```python
from build123d import *

# Parameters (mm, degrees)
SKETCH1_R                = 57.15
SKETCH1_R_2              = 53.34
SCHEDULED_CHAMBER_DEPTH  = 260.35
SKETCH2_R                = 76.2
SKETCH2_R_2              = 57.15
FLANGE_DEPTH             = 6.35
ORIGINAL_BOLT_HOLE_REACH = 283.771
SKETCH3_R                = 3.175
BOLT_HOLE_PATTERN_COUNT  = 8


with BuildPart() as part:
    # Sketch1 → Scheduled Chamber (new body)
    with BuildSketch(Plane(origin=(0, 0, 0), x_dir=(1, 0, 0), z_dir=(0, 1, 0))):
        with Locations(Location((0, 0, 0), (0, 0, 270))):
            Circle(SKETCH1_R)
        with Locations(Location((0, 0, 0), (0, 0, 270))):
            Circle(SKETCH1_R_2, mode=Mode.SUBTRACT)
    extrude(amount=-SCHEDULED_CHAMBER_DEPTH)

    # Sketch2 → Flange (add)
    with BuildSketch(Plane(origin=(0, 0, 0), x_dir=(1, 0, 0), z_dir=(0, 1, 0))):
        with Locations(Location((0, 0, 0), (0, 0, 270))):
            Circle(SKETCH2_R)
        with Locations(Location((0, 0, 0), (0, 0, 270))):
            Circle(SKETCH2_R_2, mode=Mode.SUBTRACT)
    extrude(amount=-FLANGE_DEPTH)

    # Sketch3 → Original Bolt Hole (cut, up to next)
    with BuildSketch(Plane(origin=(0, 0, 0), x_dir=(1, 0, 0), z_dir=(0, 1, 0)), mode=Mode.PRIVATE) as original_bolt_hole_sk1:
        with Locations(Location((0, 64.77, 0), (0, 0, 270))):
            Circle(SKETCH3_R)
    original_bolt_hole_tool1 = extrude(original_bolt_hole_sk1.sketch, amount=-ORIGINAL_BOLT_HOLE_REACH, mode=Mode.PRIVATE) & part.part
    original_bolt_hole = original_bolt_hole_tool1.solids().sort_by_distance((0, 0, -64.77))[0]
    add(original_bolt_hole, mode=Mode.SUBTRACT)

    # Bolt Hole Pattern: Original Bolt Hole ×8 about axis
    bolt_hole_pattern_axis = Axis((0, 0, 0), (0, 1, 0))
    for i in range(1, BOLT_HOLE_PATTERN_COUNT):
        add(original_bolt_hole.rotate(bolt_hole_pattern_axis, i * 360 / BOLT_HOLE_PATTERN_COUNT), mode=Mode.SUBTRACT)


solid = part.part
```
Here's how the part is built. I have some questions about the finished solid (model axes, mm). A direction names the side the tool comes from. Round coordinates to 2 decimals unless told otherwise and drop trailing zeros. Order: outer loops, then holes, each group sorted by start corner. A loop starts at its lowest first (then second) coordinate and runs counter-clockwise, first axis right, second up. Notation, with made-up numbers: M 54,46 L 111,46 A19 ccw 111,80 Z; hole C -8.5,-39.75 d7. An arc over 180 degrees is marked long. Use CSV: the item, a comma, the result in double quotes.
1) I want a section at C-C (z = 64.77). List the corners of the cut face in (x, y) for me (3 decimals), then the cut area to 3 significant figures.
Taken from the geometry:
outline,"M -40.141,-6.35 L -3.175,-6.35 L -3.175,0 L -40.141,0 Z; M 3.175,-6.35 L 40.141,-6.35 L 40.141,0 L 3.175,0 Z"
area,"469 mm^2"
2) If we mould it in two halves opening along Z, with no side actions, what happens to faces 1 (the flat face through (51, -6.35, -29)), 2 (the cylindrical face through (-46.367, -3.131, -60.47)), 3 (the cylindrical face through (44.585, -3.131, 42.866))? For each: pulls with the +Z half, pulls with the -Z half, needs draft (parallel to the pull), parting line crosses it, or undercut.
Taken from the geometry:
face 1,"needs draft"
face 2,"parting line crosses it"
face 3,"undercut"
3) I need wall thicknesses on line 1 along X through (y, z) = (-29, -2) (1 decimal); line 2 along X through (y, z) = (-147.5, -6.5); line 3 along Z through (x, y) = (36.5, -83). Which ranges of each line are inside material? Lowest first, please. Write a range as [from, to].
Taken from the geometry:
line 1,"[-57.1, -53.3], [53.3, 57.1]"
line 2,"[-56.78, -52.94], [52.94, 56.78]"
line 3,"[-43.98, -38.9], [38.9, 43.98]"
4) I want a section at D-D (y = -176.5). List the corners of the cut face in (x, z) for me, then the cut area to 3 significant figures.
Taken from the geometry:
outline,"C 0,0 d114.3; hole C 0,0 d106.68"
area,"1,320 mm^2"
5) I want a section at B-B (x = -64.77). List the corners of the cut face in (y, z) for me (3 decimals).
Taken from the geometry:
outline,"M -6.35,-40.141 L 0,-40.141 L 0,-3.175 L -6.35,-3.175 Z; M -6.35,3.175 L 0,3.175 L 0,40.141 L -6.35,40.141 Z"
6) I want a section at A-A (z = 0). List the corners of the cut face in (x, y) for me (3 decimals), then the cut area to 3 significant figures.
Taken from the geometry:
outline,"M -76.2,-6.35 L -67.945,-6.35 L -67.945,0 L -76.2,0 Z; M -61.595,-6.35 L -57.15,-6.35 L -57.15,-260.35 L -53.34,-260.35 L -53.34,0 L -61.595,0 Z; M 53.34,-260.35 L 57.15,-260.35 L 57.15,-6.35 L 61.595,-6.35 L 61.595,0 L 53.34,0 Z; M 67.945,-6.35 L 76.2,-6.35 L 76.2,0 L 67.945,0 Z"
area,"2,150 mm^2"
7) I'm going to push flat-ended pins straight in: P1, Ø10, axis at x = -45.8, z = -45.8, coming from the -Y side; P2, Ø5, axis at x = 64.77, z = 0, coming from the +Y side; P3, Ø6, axis at y = -92.5, z = -28, coming from the +X side; P4, Ø1.5, axis at y = -103, z = 15, coming from the +X side. Where does each tip first touch, or does it pass through?
Taken from the geometry:
P1,"y = -6.35"
P2,"through"
P3,"x = 51.39"
P4,"x = 55.34"
8) On a 3-axis mill with a long thin cutter (end or side, diameter ignored), from which of +Z, -Z, +X, -X, +Y, -Y can I reach the whole of each face in a straight line? I mean faces 4 (the cylindrical face through (-67.94, -3.13, -0.14)), 5 (the cylindrical face through (2.513, -131.572, -57.095)). Say none if no direction works.
Taken from the geometry:
face 4,"+Y, -Y"
face 5,"-Y"
